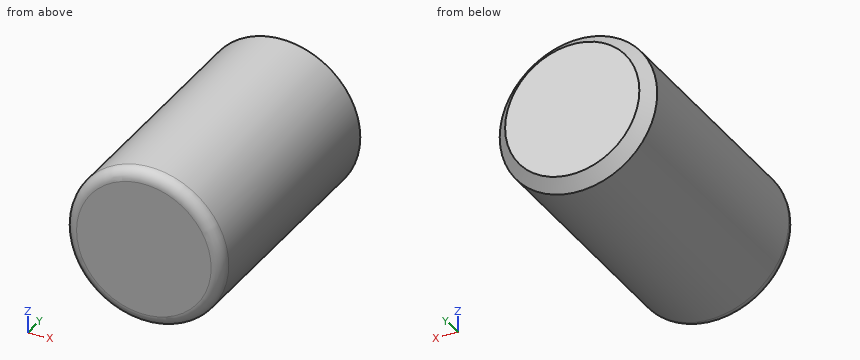
```python
from build123d import *

# Parameters (mm, degrees)
F0_R     = 34.377817
F1_DEPTH = 117.094
F2_SIZE  = 5.08
F3_R     = 5


with BuildPart() as f1:
    # F0 (on Front) → F1 (new body)
    with BuildSketch(Plane.XZ):
        Circle(F0_R)
    extrude(amount=F1_DEPTH)

    # F2
    f2_edges = [f1.edges().sort_by_distance(p)[0] for p in [
        (-34.377817, 0, 0),
    ]]
    chamfer(f2_edges, length=F2_SIZE)

    # F3
    f3_edges = [f1.edges().sort_by_distance(p)[0] for p in [
        (-34.377817, -117.094, 0),
    ]]
    fillet(f3_edges, radius=F3_R)


solid = f1.part
```
Here's how the part is built. I have some questions about the finished solid (model axes, mm). Round coordinates to 2 decimals unless told otherwise and drop trailing zeros. Write each loop counter-clockwise with the first axis right and the second up, starting at its lowest first coordinate (ties: lowest second). Pieces come first, ordered by that corner, then holes.
Q1. Will these pins go through, and if not, where does the flat tip stop? P1, Ø5, axis at x = 19, z = 27, coming from the -Y side; P2, Ø1.5, axis at y = -78, z = -17, coming from the +X side; P3, Ø8, axis at y = -29.5, z = 21.5, coming from the +X side.
Q2. If we section it at A-A on y = -57: Write out the boundary of the cut face in (x, z), plus the area to 3 significant figures.
Q3. Please list where these lines run through material, in increasing order: probe 1 along X at (y, z) = (-19, 18); probe 2 along X at (y, z) = (-44.5, -5.5) (3 decimals); probe 3 along Z at (x, y) = (25, -12.5).
Answer below:
1. P1: stops at y = -116.96
1. P2: stops at x = 30.29
1. P3: stops at x = 29.59
2. outline: circle Ø68.76 at (0, 0)
2. area: 3,710 mm2
3. probe 1: x = -29.29 to 29.29
3. probe 2: x = -33.935 to 33.935
3. probe 3: z = -23.6 to 23.6
